Verification items for the finished model (mm, model axes). A direction names the side the tool comes from. Coordinates: 2 decimals unless noted, no trailing zeros. Loops run counter-clockwise (first coordinate to the right, second up) from the corner with the lowest first, then second, coordinate; pieces in that order, holes last.
Q1. Sectioned sample at B-B (z = 0). Count the separate pieces of the cut face and the enclosed holes in it, then the cut area to 3 significant figures.
Q2. Material ranges on probe 1 along Z at (x, y) = (13, 2.6); probe 2 along X at (y, z) = (0.75, 0.5); probe 3 along Y at (x, z) = (7.5, 2.75), recorded low to high.
Q3. Access from +Z, -Z, +X, -X, +Y, -Y to the whole of each face (thin tool, end or side, straight path). Record for faces 5 (the face through (10.735, 3.338, 0.05)), 6 (the face through (16, 3, 2.266)), 7 (the face through (-2, -2.6, 0)).
Q4. Sectioned sample at D-D (y = -1). Enter the section's corners in (x, z), then the cut area to 3 significant figures.
Q5. Go/stop test with flat-tipped pins: P1, Ø5, axis at x = 16.5, z = -2.5, coming from the -Y side; P2, Ø2, axis at x = 18.5, y = 1, coming from the -Z side; P3, Ø1.4, axis at x = 16.5, y = 3.5, coming from the +Z side; P4, Ø4, axis at x = 16, z = 0, coming from the +Y side. Record where each tip stops, or that it passes through.
Q6. Mould release check, pull along Z, two halves, no side actions. Record for faces 1 (the face through (-3.905, -2.465, 0.867)), 2 (the face through (3.233, 1.317, 1.341)), 3 (the face through (10.029, 1.232, 3.344)), 4 (the face through (17.25, 2.07, -0.05)): +Z half, -Z half, draft (parallel to the pull), parting line (faces both ways), or undercut.
Q7. Sectioned sample at C-C (y = 3.5). Enter the section's corners in (x, z), then the cut area to 3 significant figures.
Q8. Sectioned sample at A-A (x = 0). Enter the section's corners in (y, z).
```python
from build123d import *

# Parameters (mm, degrees)
BOSS_EXTRU_1_DEPTH                                 = 2.5
ESQUISSE2_R                                        = 4
BOSS_EXTRU_2_DEPTH                                 = 5
ESQUISSE3_R                                        = 2.7
ENL_V_MAT_EXTRU_1_DEPTH                            = 2.4
CHAMBRAGE_POUR_VIS_T_TE_RONDE_BOMB_E_M_D           = 3.2
CHAMBRAGE_POUR_VIS_T_TE_RONDE_BOMB_E_M_CBORE_D     = 7
CHAMBRAGE_POUR_VIS_T_TE_RONDE_BOMB_E_M_CBORE_DEPTH = 2.4
BOSS_EXTRU_3_DEPTH                                 = 1.7
DIAM_TRE_DU_PER_AGE_2_5_2_5_1_D                    = 2.5


with BuildPart() as part:
    # Esquisse1 → Boss.-Extru.1 (new body)
    with BuildSketch(Plane(origin=(0, 0, 0), x_dir=(1, 0, 0), z_dir=(0, 1, 0))):
        with BuildLine():
            Line((0.529171571, 4.468778071), (19.266434362, 2.25))
            ThreePointArc((19.266434362, 2.25), (21.265720033, 0), (19.266434362, -2.25))
            Line((19.266434362, -2.25), (0.529171571, -4.468778071))
            ThreePointArc((0.529171571, -4.468778071), (-4.5, 0), (0.529171571, 4.468778071))
        make_face()
    extrude(amount=BOSS_EXTRU_1_DEPTH)

    # Esquisse2 → Boss.-Extru.2 (add)
    with BuildSketch(Plane.XZ):
        with Locations(Location((0, 0, 0), (0, 0, 270))):
            Circle(ESQUISSE2_R)
    extrude(amount=BOSS_EXTRU_2_DEPTH)

    # Esquisse3 → Enl_v. mat.-Extru.1 (cut)
    with BuildSketch(Plane.XZ.offset(5)):
        with Locations(Location((0, 0, 0), (0, 0, 270))):
            Circle(ESQUISSE3_R)
    extrude(amount=-ENL_V_MAT_EXTRU_1_DEPTH, mode=Mode.SUBTRACT)

    # Chambrage pour vis _ t_te ronde bomb_e M (through all)
    with Locations(Plane(origin=(0, 2.5, 0), x_dir=(1, 0, 0), z_dir=(0, 1, 0))):
        with Locations((0, 0)):
            CounterBoreHole(CHAMBRAGE_POUR_VIS_T_TE_RONDE_BOMB_E_M_D / 2, CHAMBRAGE_POUR_VIS_T_TE_RONDE_BOMB_E_M_CBORE_D / 2, CHAMBRAGE_POUR_VIS_T_TE_RONDE_BOMB_E_M_CBORE_DEPTH)

    # Esquisse6 → Boss.-Extru.3 (add)
    with BuildSketch(Plane(origin=(0, 2.5, 0), x_dir=(1, 0, 0), z_dir=(0, 1, 0))):
        with BuildLine():
            Line((19, -2.265720033), (13, -2.265720033))
            ThreePointArc((13, -2.265720033), (10.734279967, 0), (13, 2.265720033))
            Line((13, 2.265720033), (19, 2.265720033))
            ThreePointArc((19, 2.265720033), (21.265720033, 0), (19, -2.265720033))
        make_face()
    extrude(amount=BOSS_EXTRU_3_DEPTH)

    # Diam_tre du per_age _2.5 _2.5_1 (through all)
    with Locations(Plane(origin=(0, 4.2, 0), x_dir=(1, 0, 0), z_dir=(0, 1, 0))):
        with Locations((13, 0), (16, 0), (19, 0)):
            Hole(DIAM_TRE_DU_PER_AGE_2_5_2_5_1_D / 2)


solid = part.part
```
Geometry check:
1. separate pieces: 5
1. enclosed holes: 0
1. area: 52.4 mm2
2. probe 1: z = -2.27 to -1.25, 1.25 to 2.27
2. probe 2: x = -4.47 to -3.46, 3.46 to 11.85, 14.15 to 14.85, 17.15 to 17.85, 20.15 to 21.21
2. probe 3: y = 0 to 2.5
3. face 5: -X, +Y
3. face 6: +Z, +X, -X, +Y
3. face 7: -Y
4. outline: circle Ø8 at (0, 0); hole circle Ø3.2 at (0, 0)
4. area: 42.2 mm2
5. P1: stops at y = 0
5. P2: stops at z = -2.46
5. P3: stops at z = 2.27
5. P4: stops at y = 4.2
6. face 1: parting line
6. face 2: undercut
6. face 3: +Z half
6. face 4: undercut
7. outline: (13, -2.27) - (19, -2.27) arc R2.27 ccw to (19, 2.27) - (13, 2.27) arc R2.27 ccw to start; hole circle Ø2.5 at (13, 0); hole circle Ø2.5 at (16, 0); hole circle Ø2.5 at (19, 0)
7. area: 28.6 mm2
8. outline: (-5, -4) - (0, -4) - (0, -4.5) - (2.5, -4.5) - (2.5, -3.5) - (0.1, -3.5) - (0.1, -1.6) - (-2.6, -1.6) - (-2.6, -2.7) - (-5, -2.7) - close; (-5, 2.7) - (-2.6, 2.7) - (-2.6, 1.6) - (0.1, 1.6) - (0.1, 3.5) - (2.5, 3.5) - (2.5, 4.5) - (0, 4.5) - (0, 4) - (-5, 4) - close
